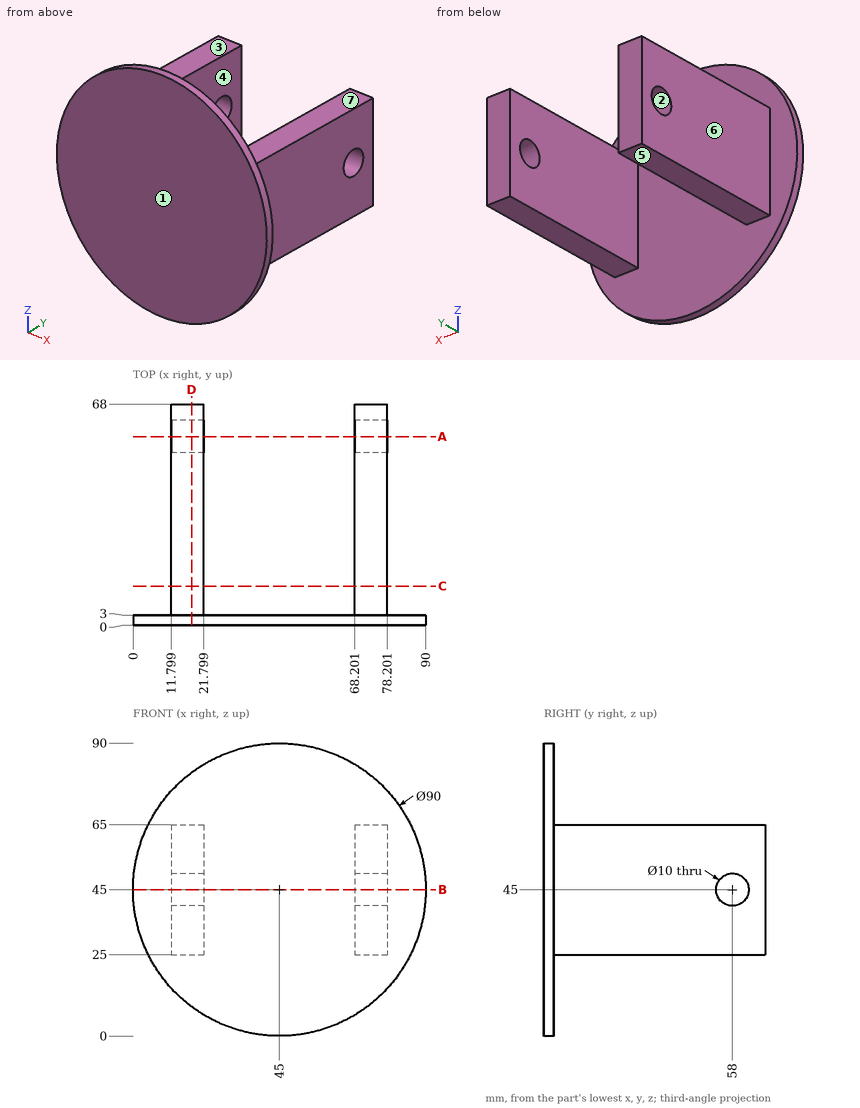
Design review of the part shown in the three views and the two pictorial views. Dimensions are in mm from the part's minimum x, y and z. A direction names the side the tool comes from. Round coordinates to 2 decimals unless told otherwise and drop trailing zeros. Write each loop counter-clockwise with the first axis right and the second up, starting at its lowest first coordinate (ties: lowest second). Pieces come first, ordered by that corner, then holes. Notation, with made-up numbers: M -17,68 L 41,68 A34 cw 41,104 Z; hole C 24,52 d9. An arc over 180 degrees is marked long. One line per item, written item: value. Start each with the question number.
1. To check wall thickness, follow probe 1 along X at (y, z) = (37.5, 38); probe 2 along Y at (x, z) = (75, 45); probe 3 along Y at (x, z) = (53, 64). State the ranges of each line that lie inside material, in increasing order. Write a range as from..to.
2. Take a section at A-A on y = 58. State the section outline as (x, z) points.
3. Take a section at D-D on x = 18. State the section outline as (y, z) points.
4. For the marked faces 4, 5, 6 and 7, list the 3-axis set-ups (+Z, -Z, +X, -X, +Y, -Y) from which the entire face can be reached by the end or side of a thin tool; tool diameter is ignored.
5. Clearance check with flat-ended pins moving along their axes: P1, Ø3, axis at x = 71, y = 43, coming from the +Z side; P2, Ø11.5, axis at y = 58, z = 45, coming from the -X side; P3, Ø5, axis at x = 71.5, y = 46.5, coming from the -Z side; P4, Ø10, axis at x = 34, y = 11.5, coming from the -Z side. State where each tip first meets the part, or that it passes through.
6. Take a section at C-C on y = 12. State the section outline as (x, z) points, then the cut area to 3 significant figures.
7. Draft analysis for pull direction Z (two halves, no side actions). For the marked faces 1, 2 and 3, state which applies: pulls with the +Z half, pulls with the -Z half, needs draft (parallel to the pull), parting line crosses it, or undercut.
8. Take a section at B-B on z = 45. State the section outline as (x, y) points.
Computed:
1. probe 1: x = 11.8..21.8, 68.2..78.2
1. probe 2: y = 0..53, 63..68
1. probe 3: y = 0..3
2. outline: M 11.8,25 L 21.8,25 L 21.8,40 L 11.8,40 Z; M 11.8,50 L 21.8,50 L 21.8,65 L 11.8,65 Z; M 68.2,25 L 78.2,25 L 78.2,40 L 68.2,40 Z; M 68.2,50 L 78.2,50 L 78.2,65 L 68.2,65 Z
3. outline: M 0,9 L 3,9 L 3,25 L 68,25 L 68,65 L 3,65 L 3,81 L 0,81 Z; hole C 58,45 d10
4. face 4: +Z, -Z, +Y
4. face 5: -Z, +X, -X, +Y
4. face 6: +Z, -Z, -X, +Y
4. face 7: +Z, +X, -X, +Y
5. P1: stops at z = 65
5. P2: stops at x = 11.8
5. P3: stops at z = 25
5. P4: passes through
6. outline: M 11.8,25 L 21.8,25 L 21.8,65 L 11.8,65 Z; M 68.2,25 L 78.2,25 L 78.2,65 L 68.2,65 Z
6. area: 800 mm²
7. face 1: needs draft
7. face 2: undercut
7. face 3: pulls with the +Z half
8. outline: M 0,0 L 90,0 L 90,3 L 78.2,3 L 78.2,53 L 68.2,53 L 68.2,3 L 21.8,3 L 21.8,53 L 11.8,53 L 11.8,3 L 0,3 Z; M 11.8,63 L 21.8,63 L 21.8,68 L 11.8,68 Z; M 68.2,63 L 78.2,63 L 78.2,68 L 68.2,68 Z
